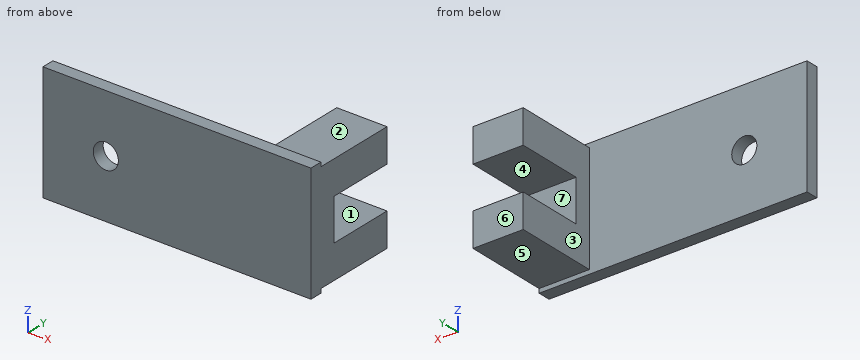
from build123d import *

# Parameters (mm, degrees)
SKETCH1_W           = 32
SKETCH1_H           = 14
SKETCH1_R           = 1.5
BOSS_EXTRUDE1_DEPTH = 1.5
SKETCH2_W           = 6
SKETCH2_H           = 13
BOSS_EXTRUDE2_DEPTH = 2
SKETCH3_W           = 6
SKETCH3_H           = 4
BOSS_EXTRUDE3_DEPTH = 8


with BuildPart() as part:
    # Sketch1 → Boss-Extrude1 (new body)
    with BuildSketch(Plane(origin=(0, 0, 0), x_dir=(1, 0, 0), z_dir=(0, 1, 0))):
        Rectangle(SKETCH1_W, SKETCH1_H)
        with Locations(Location((-8.5, 0, 0), (0, 0, 270))):
            Circle(SKETCH1_R, mode=Mode.SUBTRACT)
    extrude(amount=BOSS_EXTRUDE1_DEPTH)

    # Sketch2 → Boss-Extrude2 (add)
    with BuildSketch(Plane(origin=(0, 1.5, 0), x_dir=(1, 0, 0), z_dir=(0, 1, 0))):
        with Locations((13, 0)):
            Rectangle(SKETCH2_W, SKETCH2_H)
    extrude(amount=BOSS_EXTRUDE2_DEPTH)

    # Sketch3 → Boss-Extrude3 (add)
    with BuildSketch(Plane(origin=(0, 3.5, 0), x_dir=(1, 0, 0), z_dir=(0, 1, 0))):
        with Locations((13, 4.5)):
            Rectangle(SKETCH3_W, SKETCH3_H)
        with Locations((13, -4.5)):
            Rectangle(SKETCH3_W, SKETCH3_H)
    extrude(amount=BOSS_EXTRUDE3_DEPTH)


solid = part.part
Part model, mm, in its own coordinate system. Face numbers are marked on the shaded views. A direction names the side the tool comes from. Give positions to 0.01 mm unless a question says otherwise; leave off trailing zeros. Order: outer loops, then holes, each group sorted by start corner. A loop starts at its lowest first (then second) coordinate and runs counter-clockwise, first axis right, second up. Notation, with made-up numbers: (30.5, -32) - (76.5, -32) arc R22 cw to (76.5, -25) - close; hole circle Ø6 at (18.5, -11.75). An arc over 180 degrees is marked (long way). Use a Markdown table: item, result.
1) Two-plate mould, pull along Z, no slides. Class the marked faces 4, 5, 6 and 7: +Z half, -Z half, draft (parallel to the pull), parting line (faces both ways), or undercut.
Checked values:
| item | result |
|---|---|
| face 4 | undercut |
| face 5 | -Z half |
| face 6 | draft |
| face 7 | undercut |
2) Saw through at C-C on x = -8.5. List the corners of the cut face in (y, z), plus the area to 3 significant figures.
Checked values:
| item | result |
|---|---|
| outline | (0, -7) - (1.5, -7) - (1.5, -1.5) - (0, -1.5) - close; (0, 1.5) - (1.5, 1.5) - (1.5, 7) - (0, 7) - close |
| area | 16.5 mm² |
3) 3-axis set-ups, long thin cutter, end or side, ignore diameter. For the marked faces 1, 2 and 3: which of +Z, -Z, +X, -X, +Y, -Y reach the whole face in a straight line?
Checked values:
| item | result |
|---|---|
| face 1 | +X, -X, +Y |
| face 2 | +Z, +X, -X, +Y |
| face 3 | +Z, -Z, -X, +Y |
4) Saw through at B-B on y = 8.5. List the corners of the cut face in (x, z), plus the area to 3 significant figures.
Checked values:
| item | result |
|---|---|
| outline | (10, -6.5) - (16, -6.5) - (16, -2.5) - (10, -2.5) - close; (10, 2.5) - (16, 2.5) - (16, 6.5) - (10, 6.5) - close |
| area | 48.0 mm² |
5) Saw through at A-A on z = 0. List the corners of the cut face in (x, y), plus the area to 3 significant figures.
Checked values:
| item | result |
|---|---|
| outline | (-16, 0) - (-10, 0) - (-10, 1.5) - (-16, 1.5) - close; (-7, 0) - (16, 0) - (16, 3.5) - (10, 3.5) - (10, 1.5) - (-7, 1.5) - close |
| area | 55.5 mm² |
6) Flat gauge pins, fed straight in: P1, Ø3, axis at y = 9, z = 2.5, coming from the -X side; P2, Ø5.5, axis at x = 12, z = -1, coming from the +Y side; P3, Ø6.5, axis at x = 12.5, y = 5, coming from the +Z side; P4, Ø3, axis at x = 13, y = 6, coming from the -Z side. Where does each tip first touch, or does it go through?
Checked values:
| item | result |
|---|---|
| P1 | x = 10 |
| P2 | y = 11.5 |
| P3 | z = 6.5 |
| P4 | z = -6.5 |
7) Saw through at D-D on y = 1. List the corners of the cut face in (x, z).
Checked values:
| item | result |
|---|---|
| outline | (-16, -7) - (16, -7) - (16, 7) - (-16, 7) - close; hole circle Ø3 at (-8.5, 0) |
8) Probe L1, parallel to X at y = 0.9, z = 0; L2, parallel to Y at x = 8, z = -1; L3, parallel to X at y = 5.5, z = -4.5. List the from-to ranges inside material, lowest first. Write a range as from..to.
Checked values:
| item | result |
|---|---|
| L1 | -16..-10, -7..16 |
| L2 | 0..1.5 |
| L3 | 10..16 |
